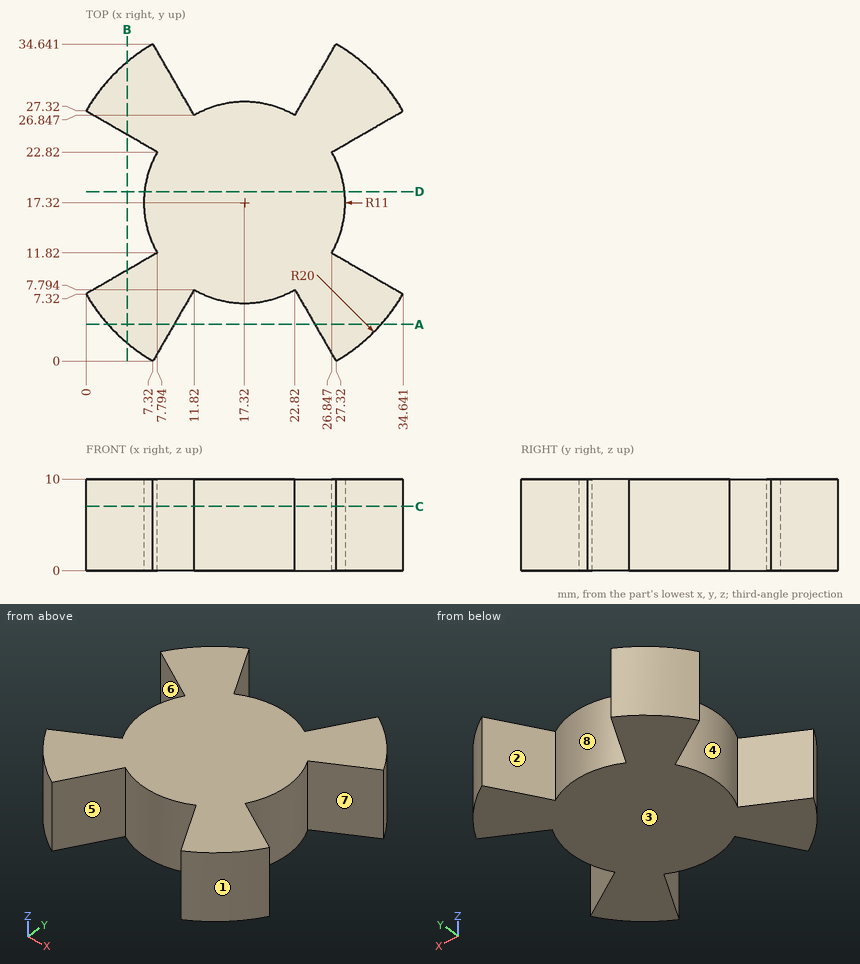
Answer from the drawing. Dimensions are ordinates in mm from the lowest x, y and z of the part. A direction names the side the tool comes from. Give positions to 0.01 mm unless a question says otherwise; leave off trailing zeros. Write each loop counter-clockwise with the first axis right and the second up, starting at its lowest first coordinate (ties: lowest second). Pieces come first, ordered by that corner, then holes. Notation, with made-up numbers: (23, 33.25) -> (35, 33.25) arc R17 cw to (35, 58.25) -> close; hole circle Ø7 at (-37.5, 34). An arc over 180 degrees is marked (long way). Use a Markdown table: item, result.
(1) For the marked faces 5, 6, 7 and 8, determine the directions among +Z, -Z, +X, -X, +Y, -Y from which every point of the face is accessible in a straight line to the end or side of a thin tool.
Return value:
| item | result |
|---|---|
| face 5 | +Z, -Z, -Y |
| face 6 | +Z, -Z, -X |
| face 7 | +Z, -Z, +X |
| face 8 | +Z, -Z, +Y |
(2) Section B-B, the plane x = 4.5 is taken. Determine the outline of the cut face in (y, z).
Return value:
| item | result |
|---|---|
| outline | (1.97, 0) -> (9.92, 0) -> (9.92, 10) -> (1.97, 10) -> close; (24.72, 0) -> (32.67, 0) -> (32.67, 10) -> (24.72, 10) -> close |
(3) Section C-C, the plane z = 7 is taken. Determine the outline of the cut face in (x, y) (1 decimal), then the cut area to 3 significant figures.
Return value:
| item | result |
|---|---|
| outline | (0, 7.3) arc R20 ccw to (7.3, 0) -> (11.8, 7.8) arc R11 ccw to (22.8, 7.8) -> (27.3, 0) arc R20 ccw to (34.6, 7.3) -> (26.8, 11.8) arc R11 ccw to (26.8, 22.8) -> (34.6, 27.3) arc R20 ccw to (27.3, 34.6) -> (22.8, 26.8) arc R11 ccw to (11.8, 26.8) -> (7.3, 34.6) arc R20 ccw to (0, 27.3) -> (7.8, 22.8) arc R11 ccw to (7.8, 11.8) -> close |
| area | 672 mm2 |
(4) Section D-D, the plane y = 18.5 is taken. Determine the outline of the cut face in (x, z).
Return value:
| item | result |
|---|---|
| outline | (6.38, 0) -> (28.26, 0) -> (28.26, 10) -> (6.38, 10) -> close |
(5) Find the intervals of material crossed by probe 1 along X at (y, z) = (17, 8.5) (1 decimal); probe 2 along X at (y, z) = (29, 4.25) (1 decimal); probe 3 along X at (y, z) = (32, 5.75) (1 decimal), in increasing order. Write a range as from..to.
Return value:
| item | result |
|---|---|
| probe 1 | 6.3..28.3 |
| probe 2 | 1.1..10.6, 24.1..33.6 |
| probe 3 | 3.7..8.8, 25.8..30.9 |
(6) Section A-A, the plane y = 4 is taken. Determine the outline of the cut face in (x, z).
Return value:
| item | result |
|---|---|
| outline | (2.4, 0) -> (9.63, 0) -> (9.63, 10) -> (2.4, 10) -> close; (25.01, 0) -> (32.24, 0) -> (32.24, 10) -> (25.01, 10) -> close |
(7) Determine the mould class of the marked faces 1, 2, 3 and 4 for opening direction Y: released by +Y, released by -Y, zero draft, split by the parting line, or undercut.
Return value:
| item | result |
|---|---|
| face 1 | released by -Y |
| face 2 | released by +Y |
| face 3 | zero draft |
| face 4 | undercut |
(8) Flat-ended cylindrical pins translate along their axes: P1, Ø1.5, axis at x = 11, z = 8, coming from the +Y side (1 decimal); P2, Ø1.5, axis at y = 10, z = 3, coming from the -X side (1 decimal); P3, Ø4, axis at x = 13, z = 8, coming from the -Y side (1 decimal); P4, Ø1.5, axis at x = 23.5, y = 30, coming from the +Z side. Find the tip coordinate at first contact, or state that the pin passes through.
Return value:
| item | result |
|---|---|
| P1 | y = 29.6 |
| P2 | x = 3.3 |
| P3 | y = 6.4 |
| P4 | through |
